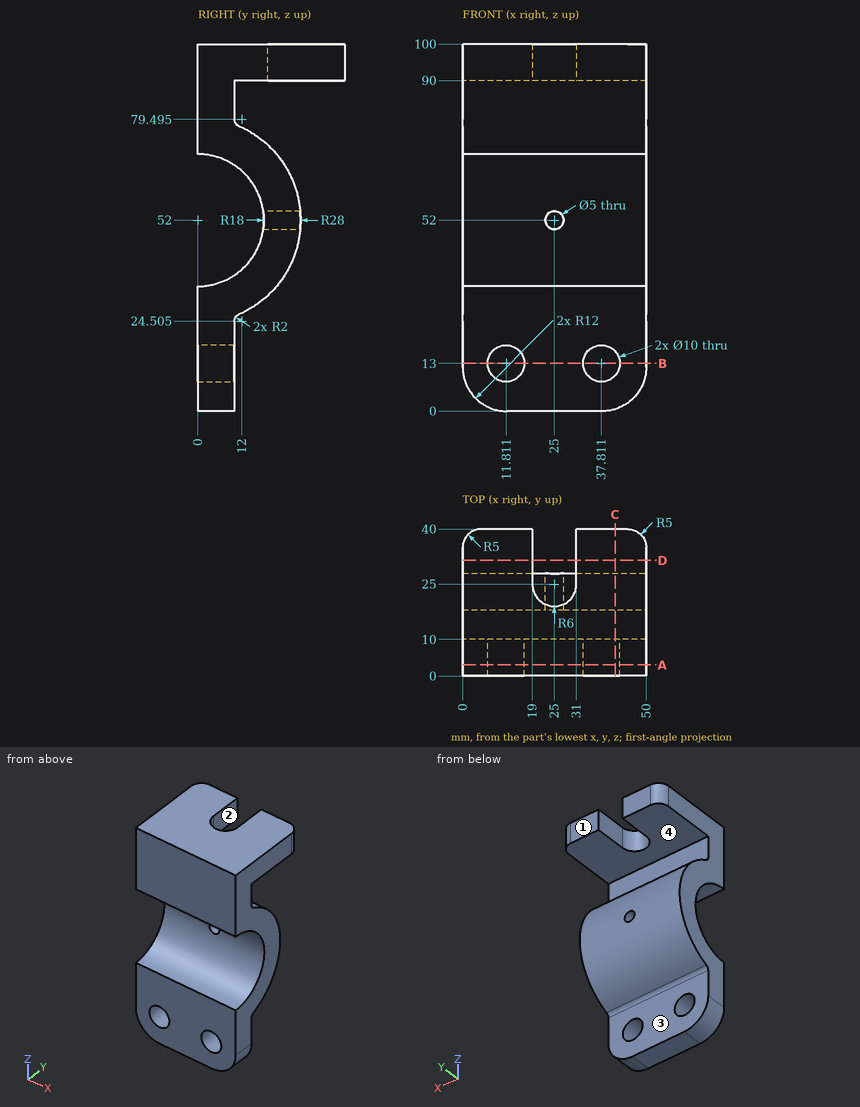
Part print with two shaded views. Sizes in mm from the minimum x, y, z corner. A direction names the side the tool comes from. Round coordinates to 2 decimals unless told otherwise and drop trailing zeros. Loops run counter-clockwise (first coordinate to the right, second up) from the corner with the lowest first, then second, coordinate; pieces in that order, holes last.
Item 1: Pin check, flat tips, straight feed: P1, Ø13, axis at x = 11.81, z = 13, coming from the +Y side; P2, Ø3, axis at x = 11, z = 38, coming from the +Y side (1 decimal); P3, Ø6, axis at x = 32.5, z = 23, coming from the +Y side; P4, Ø4.5, axis at x = 25, z = 52, coming from the -Y side. Stop position of each tip, or through.
Item 2: Drill centre lines: line 1 along X through (y, z) = (5.5, 13); line 2 along Z through (x, y) = (3, 13); line 3 along Y through (x, z) = (19, 80). Where is each one in solid material? Low to high.
Item 3: Saw through at C-C (x = 41.5). List the corners of the cut face in (y, z) (1 decimal), then the cut area to 3 significant figures.
Item 4: Which spindle directions (+Z, -Z, +X, -X, +Y, -Y) get a long thin tool onto all of the face, cutting with end or side? Do the marked faces 1, 2, 3 and 4. Say none if no direction does.
Item 5: Saw through at D-D (y = 31.5). List the corners of the cut face in (x, z), then the cut area to 3 significant figures.
Item 6: Saw through at B-B (z = 13). List the corners of the cut face in (x, y), then the cut area to 3 significant figures.
Item 7: Saw through at A-A (y = 3). List the corners of the cut face in (x, z).
Worked answers:
1. P1: stops at y = 10
1. P2: stops at y = 25.1
1. P3: stops at y = 10.67
1. P4: passes through
2. line 1: x = 0 to 6.81, 16.81 to 32.81, 42.81 to 50
2. line 2: z = 27.2 to 39.55, 64.45 to 76.8, 90 to 100
2. line 3: y = 0 to 10
3. outline: (0, 0.5) - (10, 0.5) - (10, 9.6) - (0, 9.6) - close; (0, 16.4) - (10, 16.4) - (10, 24.5) arc R2 cw to (11.2, 26.3) arc R28 ccw to (11.2, 77.7) arc R2 cw to (10, 79.5) - (10, 90) - (40, 90) - (40, 100) - (0, 100) - (0, 70) arc R18 cw to (0, 34) - close
3. area: 1,400 mm2
4. face 1: +Z, -Z, +X, -X, +Y
4. face 2: +Z, +Y
4. face 3: -Z, +X, -X, +Y
4. face 4: +X, -X, +Y
5. outline: (0, 90) - (19, 90) - (19, 100) - (0, 100) - close; (31, 90) - (50, 90) - (50, 100) - (31, 100) - close
5. area: 380 mm2
6. outline: (0, 0) - (6.81, 0) - (6.81, 10) - (0, 10) - close; (16.81, 0) - (32.81, 0) - (32.81, 10) - (16.81, 10) - close; (42.81, 0) - (50, 0) - (50, 10) - (42.81, 10) - close
6. area: 300 mm2
7. outline: (0, 12) arc R12 ccw to (12, 0) - (38, 0) arc R12 ccw to (50, 12) - (50, 34.25) - (0, 34.25) - close; (0, 69.75) - (50, 69.75) - (50, 100) - (0, 100) - close; hole circle Ø10 at (11.81, 13); hole circle Ø10 at (37.81, 13)
